Model file for the job. Use its own axes, mm. Face numbers are marked on the shaded views. A direction names the side the tool comes from. Coordinates: 2 decimals unless noted, no trailing zeros. Order: outer loops, then holes, each group sorted by start corner. A loop starts at its lowest first (then second) coordinate and runs counter-clockwise, first axis right, second up. Notation, with made-up numbers: M 26,-39.5 L 30,-39.5 A17 cw 30,-29.5 Z; hole C 11,-39 d5. An arc over 180 degrees is marked long. Return JSON: item names as keys, results as strings.
```python
from build123d import *

# Parameters (mm, degrees)
F1_DEPTH  = 1.25
F3_DEPTH  = 4
F4_R      = 7.5
F5_DEPTH  = 3
F7_DEPTH  = 2.5
F9_DEPTH  = 12.5
F10_R     = 3.75
F11_DEPTH = 6
F12_R     = 5
F13_DEPTH = 5
F14_SIZE  = 2
F16_DEPTH = 11
F17_R     = 8
F18_R     = 0.5
F19_W     = 20
F19_H     = 20
F19_W_2   = 9
F19_H_2   = 9
F20_DEPTH = 11.001
F21_R     = 0.99999
F22_W     = 20
F22_H     = 20
F22_W_2   = 14
F22_H_2   = 14
F23_DEPTH = 3


# Not quite as in the source:
# - a fillet or chamfer is up to 0.001 mm smaller than in the source, because OpenCascade refuses the exact size


with BuildPart() as f1:
    # F0 (on Top) → F1 (new body, symmetric)
    with BuildSketch(Plane.XY):
        with BuildLine():
            ThreePointArc((-2.4892601961, 26.7685185185), (-0.1158652446, 29.4973136057), (2.5, 27))
            Line((2.5, 27), (7.8501893912, 21.6498106088))
            Line((7.8501893912, 21.6498106088), (6.8018767371, 33.6320790747))
            ThreePointArc((6.8018767371, 33.6320790747), (-4.2336746433, 35.5044693553), (-9.391842346, 25.5705604779))
            Line((-9.391842346, 25.5705604779), (-5.5, 0))
            Line((-5.5, 0), (0, 0))
            Line((0, 0), (-2.4892601961, 26.7685185185))
        make_face()
    extrude(amount=F1_DEPTH, both=True)

    # F2 (on Top) → F3 (join, symmetric)
    with BuildSketch(Plane.XY):
        Polygon((-5.5, 0), (0, 0), (-2.4892601961, 26.7685185185), (-4.4892601961, 26.7685185185), align=None)
        with BuildLine():
            Line((-4.4892601961, 26.7685185185), (-2.4892601961, 26.7685185185))
            ThreePointArc((-2.4892601961, 26.7685185185), (-0.1158652446, 29.4973136057), (2.5, 27))
            Line((2.5, 27), (5.8501893912, 23.6498106088))
            Line((5.8501893912, 23.6498106088), (7.8501893912, 21.6498106088))
            Line((7.8501893912, 21.6498106088), (7.4803727359, 25.8768343213))
            Line((7.4803727359, 25.8768343213), (3.1786035286, 30.1786035286))
            ThreePointArc((3.1786035286, 30.1786035286), (-1.8266431422, 31.1073611498), (-4.4892601961, 26.7685185185))
        make_face()
        Polygon((7.8501893912, 21.6498106088), (5.8501893912, 23.6498106088), (5.8501893912, 20), (7.8501893912, 20), align=None)
    extrude(amount=F3_DEPTH, both=True)

    # F4 (on Front) → F5 (join)
    with BuildSketch(Plane.XZ):
        Circle(F4_R)
    extrude(amount=F5_DEPTH)

    # F6 (on Top) → F7 (join, symmetric)
    with BuildSketch(Plane.XY):
        Polygon((3.8501893912, 22), (3, 0), (5.5, 0), (5.3501893912, 22), align=None)
    extrude(amount=F7_DEPTH, both=True)

    # F8 (on Right) → F9 (cut, symmetric)
    with BuildSketch(Plane.YZ):
        Polygon((31.4952242196, 2.5), (31.4952242196, 4), (26.7685185185, 4), (15.4952242196, 4), (19.6164403488, 2.5), align=None)
        Polygon((26.7685185185, -4), (31.4952242196, -4), (31.4952242196, -2.5), (19.6164403488, -2.5), (15.4952242196, -4), align=None)
    extrude(amount=F9_DEPTH, both=True, mode=Mode.SUBTRACT)

    # F10 (on face) → F11 (join)
    with BuildSketch(Plane.XZ.offset(3)):
        Circle(F10_R)
    extrude(amount=F11_DEPTH)

    # F12 (on face) → F13 (join)
    with BuildSketch(Plane.XZ.offset(9)):
        Circle(F12_R)
    extrude(amount=F13_DEPTH)

    # F14
    f14_edges = [f1.edges().sort_by_distance(p)[0] for p in [
        (-5, -14, 0),
    ]]
    chamfer(f14_edges, length=F14_SIZE)

    # F15 (on face) → F16 (cut, through all)
    with BuildSketch(Plane.XZ.offset(14)):
        Polygon((1, 1), (1, 10), (-1, 10), (-1, 1), (-10, 1), (-10, -1), (-1, -1), (-1, -10), (1, -10), (1, -1), (10, -1), (10, 1), align=None)
    extrude(amount=-F16_DEPTH, mode=Mode.SUBTRACT)

    # F17
    f17_edges = [f1.edges().sort_by_distance(p)[0] for p in [
        (6.801877, 33.632079, 0),
    ]]
    fillet(f17_edges, radius=F17_R)

    # F18
    f18_edges = [f1.edges().sort_by_distance(p)[0] for p in [
        (5.850189, 20, 0),
        (7.850189, 20, 0),
        (5.350189, 22, 0),
        (3.850189, 22, 0),
        (2.5, 27, 0),
        (0, 0, 0),
        (5.5, 0, 0),
        (3, 0, 0),
        (-5.5, 0, 0),
    ]]
    fillet(f18_edges, radius=F18_R)

    # F19 (on face) → F20 (cut, through all)
    with BuildSketch(Plane.XZ.offset(3)):
        Rectangle(F19_W, F19_H)
        Rectangle(F19_W_2, F19_H_2, mode=Mode.SUBTRACT)
    extrude(amount=F20_DEPTH, mode=Mode.SUBTRACT)

    # F21 (radius 1 in the source; OpenCascade refuses exactly that, so slightly less here)
    f21_edges = [f1.edges().sort_by_distance(p)[0] for p in [
        (-2.65165, -3, -2.65165),
        (2.65165, -3, -2.65165),
        (2.65165, -3, 2.65165),
        (-2.65165, -3, 2.65165),
        (-1, -3, 2.307104),
        (1, -3, 2.307104),
        (2.307104, -3, 1),
        (-2.307104, -3, 1),
        (-2.307104, -3, -1),
        (2.307104, -3, -1),
        (-1, -3, -2.307104),
        (1, -3, -2.307104),
    ]]
    fillet(f21_edges, radius=F21_R)

    # F22 (on Front) → F23 (cut, through all)
    with BuildSketch(Plane.XZ):
        Rectangle(F22_W, F22_H)
        Rectangle(F22_W_2, F22_H_2, mode=Mode.SUBTRACT)
    extrude(amount=F23_DEPTH, mode=Mode.SUBTRACT)


solid = f1.part
```
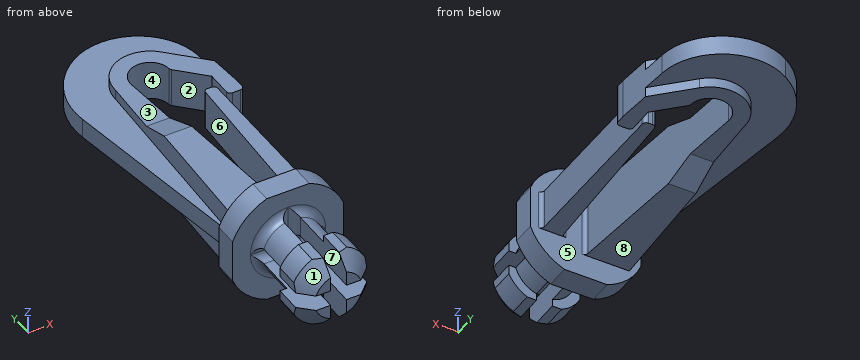
Item 1: Saw through at C-C (y = 14.5). Write the cut outline in (x, z).
Check result:
{"outline": "M -7.71,-1.25 L -4.95,-1.25 L -4.95,-4 L -1.35,-4 L -1.35,4 L -4.95,4 L -4.95,1.25 L -7.71,1.25 Z; M 3.56,-2.5 L 5.4,-2.5 L 5.4,2.5 L 3.56,2.5 Z"}
Item 2: Saw through at B-B (y = -1.5). Write the cut outline in (x, z), and give its area (3 significant figures).
Check result:
{"outline": "M -7,-2.69 A7.5 ccw -2.69,-7 L 2.69,-7 A7.5 ccw 7,-2.69 L 7,2.69 A7.5 ccw 2.69,7 L -2.69,7 A7.5 ccw -7,2.69 Z", "area": "169 mm2"}
Item 3: 3-axis set-ups, long thin cutter, end or side, ignore diameter. For the marked faces 5, 6, 7 and 8: which of +Z, -Z, +X, -X, +Y, -Y reach the whole face in a straight line?
Check result:
{"face 5": "none", "face 6": "+Z, -Z", "face 7": "+Z, -Z, -Y", "face 8": "-Z, +X, -X, +Y"}
Item 4: Wall check: line 1 (Z direction, x = 4, y = 32); line 2 (Z direction, x = 2.75, y = -8); line 3 (X direction, y = 29, z = -0.25). Give the ranges that are in metal, low to high.
Check result:
{"line 1": "z = -1.25 to 1.25", "line 2": "z = -2.55 to -1, 1 to 2.55", "line 3": "x = -9.29 to -1.5, 1.5 to 7.21"}
Item 5: Pull direction Y, two halves, no side cores. Call the marked faces 1, 2, 3 and 4: +Y half, -Y half, draft (parallel to the pull), parting line (faces both ways), or undercut.
Check result:
{"face 1": "-Y half", "face 2": "undercut", "face 3": "draft", "face 4": "undercut"}
Item 6: Saw through at D-D (z = 6.25). Write the cut outline in (x, y).
Check result:
{"outline": "M -4.15,-3 L 4.15,-3 L 4.15,0 L -4.15,0 Z"}
Item 7: Saw through at A-A (y = -8.5). Write the cut outline in (x, z).
Check result:
{"outline": "M -3.61,-1 A3.75 ccw -1,-3.61 L -1,-1 Z; M -3.61,1 L -1,1 L -1,3.61 A3.75 ccw Z; M 1,-3.61 A3.75 ccw 3.61,-1 L 1,-1 Z; M 1,1 L 3.61,1 A3.75 ccw 1,3.61 Z"}
Item 8: Drop flat-ended pins along their axis: pin 1 Ø1.8 at (x, y) = (-2.5, 7) entering from -Z; pin 2 Ø9.5 at (x, y) = (-0.5, 27.5) entering from +Z; pin 3 Ø0.5 at (x, z) = (7, 0) entering from -Y; pin 4 Ø2 at (y, z) = (-6, 5.5) entering from -X. Give the stop position or say it passes through.
Check result:
{"pin 1": "stops at z = -4", "pin 2": "stops at z = 2.5", "pin 3": "stops at y = -3", "pin 4": "passes through"}
